from build123d import *

# Parameters (mm, degrees)
ESBO_O1_R          = 4.5
FLANGE_BASE1_DEPTH = 4.8


# Sheet-metal steps are written as plain solids
with BuildPart() as part:
    # Esboço1 → Flange-base1 (new body)
    with BuildSketch(Plane(origin=(0, 0, 0), x_dir=(1, 0, 0), z_dir=(0, 1, 0))):
        with BuildLine():
            Line((-61.2, -96.2), (61.2, -96.2))
            ThreePointArc((61.2, -96.2), (68.271067812, -93.271067812), (71.2, -86.2))
            Line((71.2, -86.2), (71.2, 86.2))
            ThreePointArc((71.2, 86.2), (68.271067812, 93.271067812), (61.2, 96.2))
            Line((61.2, 96.2), (-61.2, 96.2))
            ThreePointArc((-61.2, 96.2), (-68.271067812, 93.271067812), (-71.2, 86.2))
            Line((-71.2, 86.2), (-71.2, -86.2))
            ThreePointArc((-71.2, -86.2), (-68.271067812, -93.271067812), (-61.2, -96.2))
        make_face()
        with Locations(Location((-60.6, 85.6, 0), (0, 0, 270))):
            Circle(ESBO_O1_R, mode=Mode.SUBTRACT)
        with Locations(Location((60.6, 85.6, 0), (0, 0, 270))):
            Circle(ESBO_O1_R, mode=Mode.SUBTRACT)
        with Locations(Location((-60.6, -85.6, 0), (0, 0, 270))):
            Circle(ESBO_O1_R, mode=Mode.SUBTRACT)
        with Locations(Location((60.6, -85.6, 0), (0, 0, 270))):
            Circle(ESBO_O1_R, mode=Mode.SUBTRACT)
        with Locations(Location((-20.2, 85.6, 0), (0, 0, 270))):
            Circle(ESBO_O1_R, mode=Mode.SUBTRACT)
        with Locations(Location((20.2, 85.6, 0), (0, 0, 270))):
            Circle(ESBO_O1_R, mode=Mode.SUBTRACT)
        with Locations(Location((60.6, 28.533333333, 0), (0, 0, 270))):
            Circle(ESBO_O1_R, mode=Mode.SUBTRACT)
        with Locations(Location((60.6, -28.533333333, 0), (0, 0, 270))):
            Circle(ESBO_O1_R, mode=Mode.SUBTRACT)
        with Locations(Location((20.2, -85.6, 0), (0, 0, 90))):
            Circle(ESBO_O1_R, mode=Mode.SUBTRACT)
        with Locations(Location((-20.2, -85.6, 0), (0, 0, 90))):
            Circle(ESBO_O1_R, mode=Mode.SUBTRACT)
        with Locations(Location((-60.6, -28.533333333, 0), (0, 0, 90))):
            Circle(ESBO_O1_R, mode=Mode.SUBTRACT)
        with Locations(Location((-60.6, 28.533333333, 0), (0, 0, 90))):
            Circle(ESBO_O1_R, mode=Mode.SUBTRACT)
    extrude(amount=-FLANGE_BASE1_DEPTH)


solid = part.part
Model file for the job. Use its own axes, mm. Give positions to 0.01 mm unless a question says otherwise; leave off trailing zeros. Loops run counter-clockwise (first coordinate to the right, second up) from the corner with the lowest first, then second, coordinate; pieces in that order, holes last. Notation, with made-up numbers: (20, 65) -> (40, 65) arc R14 ccw to (40, 81) -> close; hole circle Ø2 at (27, -19). An arc over 180 degrees is marked (long way). Use a Markdown table: item, result. Add a question column.
(1) Drop a flat-ended pin along its axis: pin 1 Ø8 at (x, z) = (20.2, 85.6) entering from +Y. Give the stop position or say it passes through.
(2) Slice it at A-A on x = 20.2. List the corners of the cut face in (y, z), and give its area (3 significant figures).
(3) Slice it at B-B on y = -3.85. Give the number of separate pieces and of enclosed holes in the cut face, and give its area (3 significant figures).
(4) Wall check: line 1 along X through (y, z) = (-2.2, -85.6); line 2 along Z through (x, y) = (19, -0.4); line 3 along Z through (x, y) = (18.5, -4.2). Give the ranges that are in metal, low to high.
(5) Mould opens along X. For faces 1 (the flat face through (-1, -4.8, -1)), 2 (the cylindrical face through (56.608, -2.366, -26.457)), 3 (the cylindrical face through (68.19, -2.37, 93.35)), 4 (the cylindrical face through (-56.207, -2.366, -27.558)) say: +X half, -X half, draft (parallel to the pull), parting line (faces both ways), or undercut.
Filled sheet:
| question | item | result |
|---|---|---|
| 1 | pin 1 | through |
| 2 | outline | (-4.8, -96.2) -> (0, -96.2) -> (0, -90.1) -> (-4.8, -90.1) -> close; (-4.8, -81.1) -> (0, -81.1) -> (0, 81.1) -> (-4.8, 81.1) -> close; (-4.8, 90.1) -> (0, 90.1) -> (0, 96.2) -> (-4.8, 96.2) -> close |
| 2 | area | 837 mm2 |
| 3 | separate pieces | 1 |
| 3 | enclosed holes | 12 |
| 3 | area | 26,500 mm2 |
| 4 | line 1 | -71.2 to -65.1, -56.1 to -24.7, -15.7 to 15.7, 24.7 to 56.1, 65.1 to 71.2 |
| 4 | line 2 | -96.2 to -89.94, -81.26 to 81.26, 89.94 to 96.2 |
| 4 | line 3 | -96.2 to -89.77, -81.43 to 81.43, 89.77 to 96.2 |
| 5 | face 1 | draft |
| 5 | face 2 | undercut |
| 5 | face 3 | +X half |
| 5 | face 4 | undercut |
